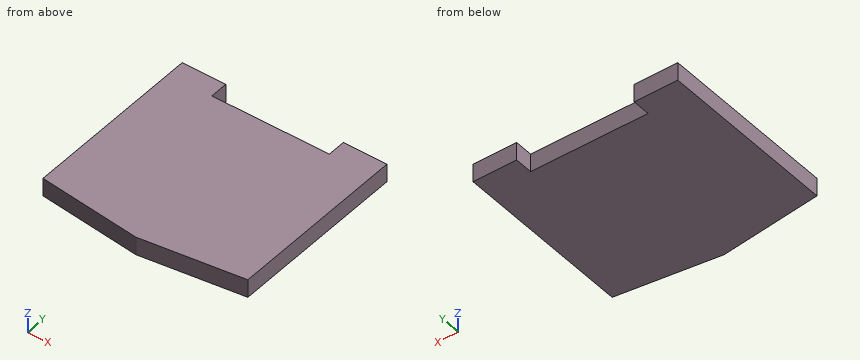
Autodesk Inventor part; units mm, degrees
ref_plane "YZ Plane" through (0, 0, 0) normal (1, 0, 0) x (0, 1, 0)
ref_plane "XZ Plane" through (0, 0, 0) normal (0, 1, 0) x (-1, 0, 0)
ref_plane "XY Plane" through (0, 0, 0) normal (0, 0, 1) x (1, 0, 0)
sketch "Sketch1" plane through (0, 0, 0) normal (0, 0, 1) x (1, 0, 0)
  line L0 (-17, 16) -> (17, 16)
  line L1 (17, 16) -> (17, -16)
  line L2 (17, -16) -> (-17, -16)
  line L3 (-17, -16) -> (-17, 16)
  line L4 (-9.75, 16) -> (9.75, 16)
  line L5 (9.75, 16) -> (9.75, 13)
  line L6 (9.75, 13) -> (-9.75, 13)
  line L7 (-9.75, 13) -> (-9.75, 16)
  line L8 (0, -16) -> (0, -13.92)
  line L9 (17, -13.92) -> (0, -16)
  line L10 (0, -16) -> (-17, -13.92)
  point P0 (0, 0)
  point P1 (17, 0)
  point P2 (0, 16)
  point P3 (9.75, 16)
  dimension "d0" = 34
  dimension "d1" = 32
  dimension "d3" = 2.08
  dimension "d6" = 19.5
  dimension "d7" = 3
extrude "Extrusion1" add sketch "Sketch1" along normal mid plane 3 contours L0 L7 L6 L5 L1 L9 L10 L3
properties part number "A"
Design review of the part built by this model. Coordinates are the model's own, in mm. Coordinates: 2 decimals unless noted, no trailing zeros. Loops run counter-clockwise (first coordinate to the right, second up) from the corner with the lowest first, then second, coordinate; pieces in that order, holes last. Notation, with made-up numbers: M 37.25,-8 L 93.25,-8 A9 cw 93.25,7 Z; hole C 54.5,41 d7. An arc over 180 degrees is marked long. Use one line per item in the form item = value.
(1) Consider section B-B (x = 9). Write out the cut boundary in (y, z).
Return value:
outline = M -14.9,-1.5 L 13,-1.5 L 13,1.5 L -14.9,1.5 Z
(2) Consider section A-A (z = 1). Write out the cut boundary in (x, y).
Return value:
outline = M -17,-13.92 L 0,-16 L 17,-13.92 L 17,16 L 9.75,16 L 9.75,13 L -9.75,13 L -9.75,16 L -17,16 Z
(3) Consider section C-C (x = -3). Write out the cut boundary in (y, z).
Return value:
outline = M -15.63,-1.5 L 13,-1.5 L 13,1.5 L -15.63,1.5 Z
(4) For line 1 along X through (y, z) = (14, 1.2); line 2 along Y through (x, z) = (9, -0.1); line 3 along Y through (x, z) = (1, -1.2), list the stretches that pass through material, from the lowest coordinate up. Write a range as from..to.
Return value:
line_1 = -17..-9.75, 9.75..17
line_2 = -14.9..13
line_3 = -15.88..13
(5) Clearance check with a flat-ended pin moving along its axis: P1, Ø0.9, axis at x = 3, z = 0.5, coming from the +Y side. State where the tip first meets the part, or that it passes through.
Return value:
P1 = 13
